```python
from build123d import *

# Parameters (mm, degrees)
SKETCH_1_W               = 340.4
SKETCH_1_H               = 900
EXTRUDE_1_DEPTH          = 292.7
SKETCH_2_R               = 22.5
CUT_EXTRUDE_1_DEPTH      = 1006.756158321
SKETCH_3_W               = 50
SKETCH_3_H               = 900
EXTRUDE_2_DEPTH          = 292.7
FILLET_9_R               = 20
FILLET_10_R              = 60
CUT_EXTRUDE_3_DEPTH      = 1024.760445612
CUT_EXTRUDE_3_DEPTH_BACK = 1024.760445612
SKETCH_5_R               = 10
CUT_EXTRUDE_4_REACH      = 1025.76
CUT_EXTRUDE_4_END_RADIUS = 22.5
SKETCH_6_R               = 15
SKETCH_7_W               = 420.4
SKETCH_7_H               = 630
CUT_EXTRUDE_6_DEPTH      = 260
CUT_EXTRUDE_7_DEPTH      = 1024.760445612


with BuildPart() as part:
    # 草图1 → 凸台-拉伸1 (new body)
    with BuildSketch(Plane.XY):
        with Locations((170.2, -450)):
            Rectangle(SKETCH_1_W, SKETCH_1_H)
    extrude(amount=EXTRUDE_1_DEPTH)

    # 草图2 → 切除-拉伸1 (cut, through all)
    with BuildSketch(Plane.XY.offset(292.7)):
        with Locations((170.2, -650)):
            Circle(SKETCH_2_R)
    extrude(amount=-CUT_EXTRUDE_1_DEPTH, mode=Mode.SUBTRACT)

    # 草图3 → 凸台-拉伸2 (add)
    with BuildSketch(Plane(origin=(0, 0, 0), x_dir=(-1, 0, 0), z_dir=(0, 0, -1))):
        with Locations((-365.4, -450)):
            Rectangle(SKETCH_3_W, SKETCH_3_H)
        with Locations((25, -450)):
            Rectangle(SKETCH_3_W, SKETCH_3_H)
    extrude(amount=-EXTRUDE_2_DEPTH)

    # 圆角9
    fillet_9_edges = [part.edges().sort_by_distance(p)[0] for p in [
        (390.4, -450, 292.7),
        (390.4, -900, 146.35),
        (390.4, 0, 146.35),
        (-50, -450, 292.7),
        (-50, 0, 146.35),
        (-50, -900, 146.35),
    ]]
    fillet(fillet_9_edges, radius=FILLET_9_R)

    # 圆角10
    # the kernel refuses this fillet: 60 mm, written as the material it takes off along each edge
    with BuildSketch(Plane(origin=(390.4, -840, 232.7), x_dir=(0, 0, 1), z_dir=(0, 1, 0))) as fillet_10_piece_1:
        with BuildLine():
            CenterArc((40, -20), 20, 0, 90)
            Line((60, -20), (60, 0))
            Line((60, 0), (40, 0))
        make_face()
    revolve(axis=Axis((390.4, -840, 232.7), (1, 0, 0)), revolution_arc=90, mode=Mode.SUBTRACT)
    with BuildSketch(Plane(origin=(-50, -840, 232.7), x_dir=(0, -1, 0), z_dir=(0, 0, -1))) as fillet_10_piece_2:
        with BuildLine():
            CenterArc((40, -20), 20, 0, 90)
            Line((60, -20), (60, 0))
            Line((60, 0), (40, 0))
        make_face()
    revolve(axis=Axis((-50, -840, 232.7), (-1, 0, 0)), revolution_arc=90, mode=Mode.SUBTRACT)
    with BuildSketch(Plane(origin=(-50, -900, 292.7), x_dir=(0, 1, 0), z_dir=(1, 0, 0))) as fillet_10_piece_3:
        with BuildLine():
            CenterArc((FILLET_10_R, -FILLET_10_R), FILLET_10_R, 90, 90)
            Line((0, -FILLET_10_R), (0, 0))
            Line((0, 0), (FILLET_10_R, 0))
        make_face()
    extrude(amount=440.4, mode=Mode.SUBTRACT)

    # 草图5 → 切除-拉伸3 (cut, two sides: drawn at the far end of the back side and taken through both)
    with BuildSketch(Plane.XY.offset(292.7).offset(-CUT_EXTRUDE_3_DEPTH_BACK)):
        with Locations((290, -440)):
            Circle(SKETCH_5_R)
    extrude(amount=CUT_EXTRUDE_3_DEPTH + CUT_EXTRUDE_3_DEPTH_BACK, mode=Mode.SUBTRACT)

    # 切除-拉伸4: up to this cylinder (the profile starts outside it)
    cut_extrude_4_end = Plane(origin=(170.2, -650, 70), z_dir=(0, 0, 1)) * Cylinder(CUT_EXTRUDE_4_END_RADIUS, 2097.52, mode=Mode.PRIVATE)
    # 草图6 → 切除-拉伸4 (cut, up to the surface)
    with BuildSketch(Plane(origin=(0, 0, 0), x_dir=(1, 0, 0), z_dir=(0, 1, 0)), mode=Mode.PRIVATE) as cut_extrude_4_sk1:
        with Locations(Location((170.2, -70, 0), (0, 0, 270))):
            Circle(SKETCH_6_R)
    cut_extrude_4_tool1 = extrude(cut_extrude_4_sk1.sketch, amount=-CUT_EXTRUDE_4_REACH, mode=Mode.PRIVATE) - cut_extrude_4_end
    add(cut_extrude_4_tool1.solids().sort_by_distance((170.2, 0, 70))[0], mode=Mode.SUBTRACT)

    # 草图7 → 切除-拉伸6 (cut)
    with BuildSketch(Plane(origin=(0, 0, 0), x_dir=(-1, 0, 0), z_dir=(0, 0, -1))):
        with Locations((-170.2, -575)):
            Rectangle(SKETCH_7_W, SKETCH_7_H)
    extrude(amount=-CUT_EXTRUDE_6_DEPTH, mode=Mode.SUBTRACT)

    # 草图8 → 切除-拉伸7 (cut, through all)
    with BuildSketch(Plane.XY.offset(292.7)):
        Polygon((170.2, -10), (0, -10), (0, -260), (340.4, -260), (340.4, -10), align=None)
    extrude(amount=-CUT_EXTRUDE_7_DEPTH, mode=Mode.SUBTRACT)


solid = part.part
```
Here's how the part is built. I have some questions about the finished solid (model axes, mm). A direction names the side the tool comes from. Coordinates: 2 decimals unless noted, no trailing zeros. Write each loop counter-clockwise with the first axis right and the second up, starting at its lowest first coordinate (ties: lowest second). Pieces come first, ordered by that corner, then holes. Notation, with made-up numbers: (36.5, -5) - (87.5, -5) arc R19 cw to (87.5, 2) - close; hole circle Ø4 at (13.25, 37.5). An arc over 180 degrees is marked (long way). One line per item, written item: value.
1) Suppose I cut it at C-C on z = 218. Write out the boundary of the cut face in (x, y), and give its area (3 significant figures).
Model answer:
outline: (-50, -880) arc R20 ccw to (-30, -900) - (370.4, -900) arc R20 ccw to (390.4, -880) - (390.4, -20) arc R20 ccw to (370.4, 0) - (-30, 0) arc R20 ccw to (-50, -20) - close; hole (-40, -890) - (380.4, -890) - (380.4, -260) - (340.4, -260) - (340.4, -10) - (0, -10) - (0, -260) - (-40, -260) - close
area: 46,100 mm²
2) We'd pull the mould along X, two halves only. Please class faces 5 (the flat face through (173, -507, 292.7)), 6 (the cylindrical face through (153.62, -634.79, 276.58)), 7 (the flat face through (-50, -456, 134)): pulls with the +X half, pulls with the -X half, needs draft (parallel to the pull), parting line crosses it, or undercut.
Model answer:
face 5: needs draft
face 6: undercut
face 7: pulls with the -X half
3) Suppose I cut it at B-B on x = 255.5. Write out the boundary of the cut face in (y, z), and give its area (3 significant figures).
Model answer:
outline: (-900, 0) - (-890, 0) - (-890, 260) - (-260, 260) - (-260, 292.7) - (-840, 292.7) arc R60 ccw to (-900, 232.7) - close; (-10, 0) - (0, 0) - (0, 292.7) - (-10, 292.7) - close
area: 25,700 mm²
4) On a 3-axis mill with a long thin cutter (end or side, diameter ignored), from which of +Z, -Z, +X, -X, +Y, -Y can I reach the whole of each face in a straight line? I mean faces 1 (the cylindrical face through (167.4, -881.96, 275.59)), 2 (the cylindrical face through (155.557, -4.93, 66.748)), 3 (the flat face through (361, -260, 128)), 4 (the flat face through (168, -260, 277)). Say none if no direction works.
Model answer:
face 1: +Z, +X, -X, -Y
face 2: +Y
face 3: -Z
face 4: +Z, -Z
5) I'm going to push a flat-ended pin straight in: P1, Ø5, axis at x = 234.5, y = -300.5, coming from the -Z side. Where does the tip first touch, or does it pass through?
Model answer:
P1: stops at z = 260
6) Suppose I cut it at A-A on y = -650. Write out the boundary of the cut face in (x, z).
Model answer:
outline: (-50, 0) - (-40, 0) - (-40, 260) - (147.7, 260) - (147.7, 292.7) - (-30, 292.7) arc R20 ccw to (-50, 272.7) - close; (192.7, 260) - (380.4, 260) - (380.4, 0) - (390.4, 0) - (390.4, 272.7) arc R20 ccw to (370.4, 292.7) - (192.7, 292.7) - close
7) I need wall thicknesses on line 1 along Y through (x, z) = (62.5, 94.5); line 2 along X through (y, z) = (-639.5, 212.5); line 3 along Y through (x, z) = (-11, 211.5). Which ranges of each line are inside material? Lowest first, please.
Model answer:
line 1: y = -900 to -890, -10 to 0
line 2: x = -50 to -40, 380.4 to 390.4
line 3: y = -900 to -890, -260 to 0
8) Suppose I cut it at D-D on x = -16.5. Write out the boundary of the cut face in (y, z).
Model answer:
outline: (-900, 0) - (-890, 0) - (-890, 260) - (-260, 260) - (-260, 0) - (0, 0) - (0, 292.7) - (-840, 292.7) arc R60 ccw to (-900, 232.7) - close
